```python
from build123d import *

# Parameters (mm, degrees)
SKETCH1_W           = 10
SKETCH1_H           = 115
BOSS_EXTRUDE1_DEPTH = 22
SKETCH3_R           = 2.05
CUT_EXTRUDE1_DEPTH  = 22
SKETCH4_R           = 3.5
CUT_EXTRUDE2_DEPTH  = 12
SKETCH7_R           = 1.75
CUT_EXTRUDE3_DEPTH  = 23


with BuildPart() as part:
    # Sketch1 → Boss-Extrude1 (new body)
    with BuildSketch(Plane(origin=(0, 0, 0), x_dir=(1, 0, 0), z_dir=(0, 1, 0))):
        Rectangle(SKETCH1_W, SKETCH1_H)
    extrude(amount=BOSS_EXTRUDE1_DEPTH)

    # Sketch3 → Cut-Extrude1 (cut)
    with BuildSketch(Plane(origin=(0, 22, 0), x_dir=(1, 0, 0), z_dir=(0, 1, 0))):
        with Locations((0, -52.5)):
            Circle(SKETCH3_R)
        with Locations((0, -2.5)):
            Circle(SKETCH3_R)
    extrude(amount=-CUT_EXTRUDE1_DEPTH, mode=Mode.SUBTRACT)

    # Sketch4 → Cut-Extrude2 (cut)
    with BuildSketch(Plane(origin=(0, 22, 0), x_dir=(1, 0, 0), z_dir=(0, 1, 0))):
        with Locations((0, -52.5)):
            Circle(SKETCH4_R)
        with Locations((0, -2.5)):
            Circle(SKETCH4_R)
    extrude(amount=-CUT_EXTRUDE2_DEPTH, mode=Mode.SUBTRACT)

    # Sketch7 → Cut-Extrude3 (cut, through all)
    with BuildSketch(Plane(origin=(0, 22, 0), x_dir=(1, 0, 0), z_dir=(0, 1, 0))):
        with Locations((0, 52.5)):
            Circle(SKETCH7_R)
        with Locations((0, 27.5)):
            Circle(SKETCH7_R)
    extrude(amount=-CUT_EXTRUDE3_DEPTH, mode=Mode.SUBTRACT)


solid = part.part
```
Could you check a few things on this model? Use its own coordinates, in mm. A direction names the side the tool comes from. Give positions to 0.01 mm unless a question says otherwise; leave off trailing zeros. Loops run counter-clockwise (first coordinate to the right, second up) from the corner with the lowest first, then second, coordinate; pieces in that order, holes last. Notation, with made-up numbers: (-39, 61.25) -> (-27, 61.25) arc R10 ccw to (-27, 66.25) -> close; hole circle Ø8 at (-25.75, -24.5). An arc over 180 degrees is marked (long way). Put each result on its own line as item: value.
(1) Imagine slicing it at B-B on z = -52.5. Write out the boundary of the cut face in (x, y).
Computed:
outline: (-5, 0) -> (-1.75, 0) -> (-1.75, 22) -> (-5, 22) -> close; (1.75, 0) -> (5, 0) -> (5, 22) -> (1.75, 22) -> close
(2) I'm going to push flat-ended pins straight in: pin 1 Ø3 at (x, z) = (0, -27.5) entering from -Y; pin 2 Ø4.5 at (x, z) = (0, 2.5) entering from +Y. Where does each tip first touch, or does it pass through?
Computed:
pin 1: through
pin 2: y = 10
(3) For faces 1 (the face through (2, 10, 54)), 2 (the face through (0, 0, -1)), which set-ups out of +Z, -Z, +X, -X, +Y, -Y let a thin tool reach every point of the face, with its end or its side?
Computed:
face 1: +Y
face 2: +Z, -Z, +X, -X, -Y
(4) Imagine slicing it at D-D on z = 52.5. Write out the boundary of the cut face in (x, y), plus the area to 3 significant figures.
Computed:
outline: (-5, 0) -> (-2.05, 0) -> (-2.05, 10) -> (-3.5, 10) -> (-3.5, 22) -> (-5, 22) -> close; (2.05, 0) -> (5, 0) -> (5, 22) -> (3.5, 22) -> (3.5, 10) -> (2.05, 10) -> close
area: 95.0 mm^2
(5) Imagine slicing it at C-C on y = 5.25. Write out the boundary of the cut face in (x, z).
Computed:
outline: (-5, -57.5) -> (5, -57.5) -> (5, 57.5) -> (-5, 57.5) -> close; hole circle Ø4.1 at (0, 2.5); hole circle Ø4.1 at (0, 52.5); hole circle Ø3.5 at (0, -52.5); hole circle Ø3.5 at (0, -27.5)
(6) Imagine slicing it at A-A on x = 0. Write out the boundary of the cut face in (y, z).
Computed:
outline: (0, -57.5) -> (22, -57.5) -> (22, -54.25) -> (0, -54.25) -> close; (0, -50.75) -> (22, -50.75) -> (22, -29.25) -> (0, -29.25) -> close; (0, -25.75) -> (22, -25.75) -> (22, -1) -> (10, -1) -> (10, 0.45) -> (0, 0.45) -> close; (0, 4.55) -> (10, 4.55) -> (10, 6) -> (22, 6) -> (22, 49) -> (10, 49) -> (10, 50.45) -> (0, 50.45) -> close; (0, 54.55) -> (10, 54.55) -> (10, 56) -> (22, 56) -> (22, 57.5) -> (0, 57.5) -> close
(7) Please list where these lines run through material, in increasing order: probe 1 along Z at (x, y) = (0, 3.25); probe 2 along Z at (x, y) = (0, 15.25); probe 3 along X at (y, z) = (17.5, 52.5). Write a range as [from, to].
Computed:
probe 1: [-57.5, -54.25], [-50.75, -29.25], [-25.75, 0.45], [4.55, 50.45], [54.55, 57.5]
probe 2: [-57.5, -54.25], [-50.75, -29.25], [-25.75, -1], [6, 49], [56, 57.5]
probe 3: [-5, -3.5], [3.5, 5]
(8) Thinking about a two-plate mould opening in X: for faces 3 (the face through (0, 11, -57.5)), 4 (the face through (-0.267, 5.07, 50.467)), 5 (the face through (5, 11, 1)), which applies, pulls with the +X half, pulls with the -X half, needs draft (parallel to the pull), parting line crosses it, or undercut?
Computed:
face 3: needs draft
face 4: undercut
face 5: pulls with the +X half
